from build123d import *

# Parameters (mm, degrees)
CYLINDER244_R           = 5.5
CYLINDER244_DEPTH       = 5
CYLINDER243_R           = 12.5
CYLINDER243_DEPTH       = 10
CYLINDER242_R           = 5
CYLINDER242_DEPTH       = 59
CYLINDER242_PITCH_ANGLE = 90
BOX124_W                = 23
BOX124_H                = 40
BOX124_DEPTH            = 87
BOX123_W                = 59
BOX123_H                = 40
BOX123_DEPTH            = 137
CUT269_PLACEMENT_ANGLE  = 90
FILLET_R                = 3


with BuildPart() as cilindro139:
    # Cylinder244 → Cylinder244 (new body)
    with BuildSketch(Plane(origin=(30, 15, 122), x_dir=(1, 0, 0), z_dir=(0, 0, 1))):
        Circle(CYLINDER244_R)
    extrude(amount=CYLINDER244_DEPTH)


with BuildPart() as cilindro138:
    # Cylinder243 → Cylinder243 (new body)
    with BuildSketch(Plane(origin=(30, 15, 127), x_dir=(1, 0, 0), z_dir=(0, 0, 1))):
        Circle(CYLINDER243_R)
    extrude(amount=CYLINDER243_DEPTH)


with BuildPart() as cilindro137:
    # Cylinder242 → Cylinder242 (new body)
    with BuildSketch(Plane.XY):
        Circle(CYLINDER242_R)
    extrude(amount=CYLINDER242_DEPTH)


with BuildPart() as cilindro137_1:
    # Cylinder242 pitch: moved
    add(cilindro137.part.rotate(Axis((0, 0, 0), (0, 1, 0)), CYLINDER242_PITCH_ANGLE))


with BuildPart() as cilindro137_2:
    # Cylinder242 placement: moved
    add(cilindro137_1.part.moved(Location((0, 15, 22))))


with BuildPart() as cubo086:
    # Box124 → Box124 (new body)
    with BuildSketch(Plane(origin=(18, -5, 0), x_dir=(1, 0, 0), z_dir=(0, 0, 1))):
        with Locations((11.5, 20)):
            Rectangle(BOX124_W, BOX124_H)
    extrude(amount=BOX124_DEPTH)


with BuildPart() as fillet_body:
    # Box123 → Box123 (new body)
    with BuildSketch(Plane(origin=(0, -5, 0), x_dir=(1, 0, 0), z_dir=(0, 0, 1))):
        with Locations((29.5, 20)):
            Rectangle(BOX123_W, BOX123_H)
    extrude(amount=BOX123_DEPTH)

    # Cut266: cut Cubo086
    add(cubo086.part, mode=Mode.SUBTRACT)

    # Cut267: cut Cilindro137
    add(cilindro137_2.part, mode=Mode.SUBTRACT)

    # Cut268: cut Cilindro138
    add(cilindro138.part, mode=Mode.SUBTRACT)

    # Cut269: cut Cilindro139
    add(cilindro139.part, mode=Mode.SUBTRACT)


with BuildPart() as fillet_body_1:
    # Cut269 placement: moved
    add(fillet_body.part.moved(Location((-444, 431, -153))).rotate(Axis((-444, 431, -153), (0, 0, 1)), CUT269_PLACEMENT_ANGLE))

    # Fillet
    fillet_edges = [fillet_body_1.edges().sort_by_distance(p)[0] for p in [
        (-459, 431, -16),
        (-459, 490, -16),
    ]]
    fillet(fillet_edges, radius=FILLET_R)


solid = fillet_body_1.part
The listing builds one solid part. Answer for the finished solid, in the listing's coordinates (mm). A direction names the side the tool comes from. Round coordinates to 2 decimals unless told otherwise and drop trailing zeros. Order: outer loops, then holes, each group sorted by start corner. A loop starts at its lowest first (then second) coordinate and runs counter-clockwise, first axis right, second up. Notation, with made-up numbers: M 49.25,49.5 L 55.25,49.5 A25 cw 55.25,72.5 Z; hole C 4,24.25 d10. An arc over 180 degrees is marked long. Answer in a Markdown table with one row per item. Add a question column.
1) The part is cut by section C-C on z = -82.5. Determine the outline of the cut face in (x, y).
2) Flat-ended cylindrical pins translate along their axes: pin 1 Ø9 at (x, y) = (-456.5, 463) entering from +Z; pin 2 Ø11.5 at (x, y) = (-455.5, 464.5) entering from -Z; pin 3 Ø6.5 at (x, y) = (-459, 461) entering from +Z. Find the tip coordinate at first contact, or state that the pin passes through.
3) Which of the six approach directions +Z, -Z, +X, -X, +Y, -Y give full straight-line access (tool end or side, diameter ignored) to faces 4 (the face through (-459.55, 448.512, -21.07)), 5 (the face through (-459, 449, -110)), 6 (the face through (-463, 481, -134))?
4) Consider line 1 along Y through (x, z) = (-446, -92); line 2 along X through (y, z) = (485.75, -131); line 3 along X through (y, z) = (461, -29). Determine where each line is inside the solid, lowest interval first. Write a range as from..to.
5) The part is cut by section A-A on z = -131. Determine the outline of the cut face in (x, y), plus the area to 3 significant figures.
6) The part is cut by section B-B on x = -459. Determine the outline of the cut face in (y, z), plus the area to 3 significant figures.
7) The part is cut by section D-D on y = 461. Determine the outline of the cut face in (x, z).
8) Determine the mould class of faces 1 (the face through (-454, 464, -26)), 2 (the face through (-459, 440, -153)), 3 (the face through (-439, 473, -85)) for opening direction X: pulls with the +X half, pulls with the -X half, needs draft (parallel to the pull), parting line crosses it, or undercut.
Findings below:
| question | item | result |
|---|---|---|
| 1 | outline | M -479,431 L -439,431 L -439,449 L -479,449 Z; M -479,472 L -439,472 L -439,490 L -479,490 Z |
| 2 | pin 1 | stops at z = -26 |
| 2 | pin 2 | stops at z = -66 |
| 2 | pin 3 | stops at z = -31 |
| 3 | face 4 | +Z |
| 3 | face 5 | -Z, +X, -X |
| 3 | face 6 | +Y, -Y |
| 4 | line 1 | y = 431..449, 472..490 |
| 4 | line 2 | x = -479..-464, -454..-439 |
| 4 | line 3 | x = -479..-464.5, -453.5..-439 |
| 5 | outline | M -479,431 L -464,431 L -464,449 L -479,449 Z; M -479,472 L -464,472 L -464,490 L -479,490 Z; M -454,431 L -439,431 L -439,449 L -454,449 Z; M -454,472 L -439,472 L -439,490 L -454,490 Z |
| 5 | area | 1,080 mm² |
| 6 | outline | M 431,-153 L 449,-153 L 449,-136 L 431,-136 Z; M 431,-126 L 449,-126 L 449,-66 L 472,-66 L 472,-126 L 490,-126 L 490,-19 A3 ccw 487,-16 L 473.5,-16 L 473.5,-26 L 466.5,-26 L 466.5,-31 L 455.5,-31 L 455.5,-26 L 448.5,-26 L 448.5,-16 L 434,-16 A3 ccw 431,-19 Z; M 472,-153 L 490,-153 L 490,-136 L 472,-136 Z |
| 6 | area | 5,410 mm² |
| 7 | outline | M -479,-66 L -439,-66 L -439,-16 L -446.5,-16 L -446.5,-26 L -453.5,-26 L -453.5,-31 L -464.5,-31 L -464.5,-26 L -471.5,-26 L -471.5,-16 L -479,-16 Z |
| 8 | face 1 | undercut |
| 8 | face 2 | needs draft |
| 8 | face 3 | pulls with the +X half |
